The model under review builds one solid part; all positions refer to its coordinate system, in mm. Face numbers are marked on the shaded views. Coordinates: 2 decimals unless noted, no trailing zeros. Order: outer loops, then holes, each group sorted by start corner. A loop starts at its lowest first (then second) coordinate and runs counter-clockwise, first axis right, second up. Notation, with made-up numbers: M 87,84 L 143,84 A20 cw 143,91 Z; hole C 50.25,41 d11. An arc over 180 degrees is marked long. Write each question's results on one line, items separated by ' | '.
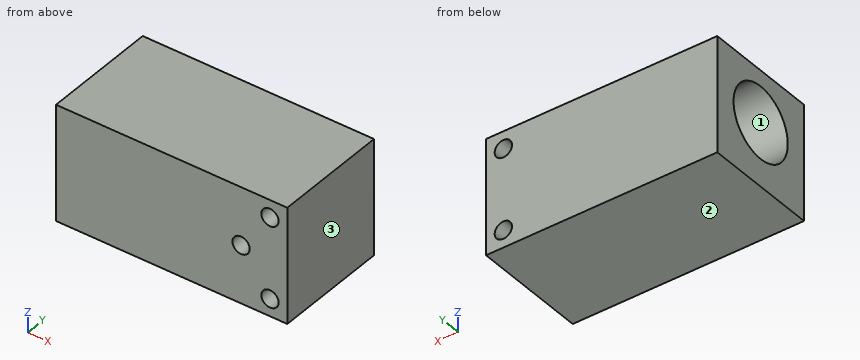
from build123d import *

# Parameters (mm, degrees)
F0_W          = 40
F0_H          = 20
F1_DEPTH      = 10
F1_DEPTH_BACK = 10
F2_R          = 6.25
F3_DEPTH      = 34
F4_R          = 1.5
F5_DEPTH      = 20.001
F6_R          = 1.5
F7_DEPTH      = 4.2727804813


with BuildPart() as f1:
    # F0 (on Front) → F1 (new body, two sides)
    with BuildSketch(Plane.XZ) as f1_sk:
        Rectangle(F0_W, F0_H)
    extrude(amount=F1_DEPTH)
    extrude(f1_sk.sketch, amount=-F1_DEPTH_BACK)

    # F2 (on face) → F3 (cut)
    with BuildSketch(Plane(origin=(-20, 0, 0), x_dir=(0, -1, 0), z_dir=(-1, 0, 0))):
        with Locations((0, 1)):
            Circle(F2_R)
    extrude(amount=-F3_DEPTH, mode=Mode.SUBTRACT)

    # F4 (on face) → F5 (cut, through all)
    with BuildSketch(Plane.XZ.offset(10)):
        with Locations((17, 7)):
            Circle(F4_R)
        with Locations((17, -7)):
            Circle(F4_R)
    extrude(amount=-F5_DEPTH, mode=Mode.SUBTRACT)

    # F6 (on face) → F7 (cut, through all)
    with BuildSketch(Plane.XZ.offset(10)):
        with Locations((12, 0)):
            Circle(F6_R)
    extrude(amount=-F7_DEPTH, mode=Mode.SUBTRACT)


solid = f1.part
1) Take a section at A-A on y = 0. State the section outline as (x, z) points, plus the area to 3 significant figures.
Solutions:
outline: M -20,-10 L 20,-10 L 20,10 L -20,10 L -20,7.25 L 14,7.25 L 14,-5.25 L -20,-5.25 Z; hole C 17,-7 d3; hole C 17,7 d3 | area: 361 mm2
2) To check wall thickness, follow line 1 along Z through (x, y) = (17, -3.25); line 2 along X through (y, z) = (-9.05, 0); line 3 along Z through (x, y) = (-13, 0). State the ranges of each line that lie inside material, in increasing order.
Solutions:
line 1: -10 to -8.5, -5.5 to 5.5, 8.5 to 10 | line 2: -20 to 10.5, 13.5 to 20 | line 3: -10 to -5.25, 7.25 to 10
3) Take a section at B-B on z = -7. State the section outline as (x, y) points, plus the area to 3 significant figures.
Solutions:
outline: M -20,-10 L 15.5,-10 L 15.5,10 L -20,10 Z; M 18.5,-10 L 20,-10 L 20,10 L 18.5,10 Z | area: 740 mm2
4) The part is to be moulded in two halves that separate along Z. For the marked faces 1, 2 and 3, say which applies: pulls with the +Z half, pulls with the -Z half, needs draft (parallel to the pull), parting line crosses it, or undercut.
Solutions:
face 1: undercut | face 2: pulls with the -Z half | face 3: needs draft
5) For pin 1 (10 mm diameter, centred on y = 3, z = 0, fed in from -X); pin 2 (11 mm diameter, centred on y = 0, z = 1, fed in from -X), all flat-tipped, find the tip position at first contact; note any pin that passes through.
Solutions:
pin 1: x = -20 | pin 2: x = 14
6) Take a section at C-C on x = -10.5. State the section outline as (y, z) points, plus the area to 3 significant figures.
Solutions:
outline: M -10,-10 L 10,-10 L 10,10 L -10,10 Z; hole C 0,1 d12.5 | area: 277 mm2
7) Take a section at D-D on y = -5. State the section outline as (x, z) points, plus the area to 3 significant figures.
Solutions:
outline: M -20,-10 L 20,-10 L 20,10 L -20,10 L -20,4.75 L 14,4.75 L 14,-2.75 L -20,-2.75 Z; hole C 17,-7 d3; hole C 17,7 d3 | area: 531 mm2
